Here's how the part is built. I have some questions about the finished solid (model axes, mm). A direction names the side the tool comes from. Round coordinates to 2 decimals unless told otherwise and drop trailing zeros. Write each loop counter-clockwise with the first axis right and the second up, starting at its lowest first coordinate (ties: lowest second). Pieces come first, ordered by that corner, then holes. Notation, with made-up numbers: (-0.75, 77) - (33.25, 77) arc R14 cw to (33.25, 88) - close; hole circle Ø9 at (-9, 76.5). An arc over 180 degrees is marked (long way). One line per item, written item: value. Start each with the question number.
Item 1: If I drill on line 1 (Z direction, x = -3.25, y = 0.75); line 2 (Z direction, x = -3.75, y = 4.25); line 3 (Y direction, x = 0, z = -14.5), over which ranges is the centre line in solid material (lowest first)?
Item 2: For P1, Ø6, axis at x = -4, z = -11.5, coming from the +Y side; P2, Ø1.2, axis at y = -2, z = 17, coming from the +X side; P3, Ø1, axis at x = -0.5, z = 2, coming from the +Y side, each with a flat end and sliding along its axis, tell me the tip position at first contact or that it passes through.
Item 3: Thinking about a two-plate mould opening in X: for faces 1 (the face through (-2.539, -1.947, 9.806)), 2 (the face through (-3, -3, 13.75)), 3 (the face through (-0.75, 0, 17)), 4 (the face through (0, 0, 16.65)), which applies, released by +X, released by -X, zero draft, split by the parting line, or undercut?
Item 4: For faces 5 (the face through (5.96, 1.88, 4.96)), 6 (the face through (3, 0, 18.15)), 7 (the face through (0.75, 0, 17)), 8 (the face through (-2.87, 2.64, -6.6)), 9 (the face through (3, -3, 5.75)), which set-ups out of +Z, -Z, +X, -X, +Y, -Y let a thin tool reach every point of the face, with its end or its side?
Item 5: Imagine slicing it at B-B, the plane x = 0. Please give me the cut outline in (y, z).
Item 6: Imagine slicing it at C-C, the plane y = 0. Please give me the cut outline in (x, z).
Item 7: Imagine slicing it at D-D, the plane z = 10. Please give me the cut outline in (x, y), then the cut area to 3 significant figures.
Item 8: Imagine slicing it at A-A, the plane y = 5. Please give me the cut outline in (x, z).
```python
from build123d import *

# Parameters (mm, degrees)
F2_W     = 1.5
F2_H     = 13
F3_DEPTH = 1.5


with BuildPart() as f1:
    # F0 (on Front) → F1 (revolve)
    with BuildSketch(Plane.XZ):
        Polygon((0, 18.15), (0, -18.15), (3.4, -18.15), (3.9, -17.65), (3.9, 4.15), (6.25, 4.15), (6.25, 5.75), (3.2, 5.75), (3.2, 13.75), (6.25, 13.75), (6.25, 18.15), align=None)
    revolve(axis=Axis((0, 0, 0), (0, 0, 1)))

    # F2 (on face) → F3 (cut)
    with BuildSketch(Plane.XY.offset(18.15)):
        Rectangle(F2_W, F2_H)
    extrude(amount=-F3_DEPTH, mode=Mode.SUBTRACT)


solid = f1.part
```
Values follow:
1. line 1: z = -18.15 to 5.75, 13.75 to 18.15
1. line 2: z = 4.15 to 5.75, 13.75 to 18.15
1. line 3: y = -3.9 to 3.9
2. P1: stops at y = 3.77
2. P2: stops at x = 6.09
2. P3: stops at y = 3.9
3. face 1: split by the parting line
3. face 2: zero draft
3. face 3: undercut
3. face 4: undercut
4. face 5: +Z, -Z
4. face 6: +Z, +X, -X, +Y, -Y
4. face 7: +Z, +Y, -Y
4. face 8: -Z
4. face 9: none
5. outline: (-6.25, 4.15) - (-3.9, 4.15) - (-3.9, -17.65) - (-3.4, -18.15) - (3.4, -18.15) - (3.9, -17.65) - (3.9, 4.15) - (6.25, 4.15) - (6.25, 5.75) - (3.2, 5.75) - (3.2, 13.75) - (6.25, 13.75) - (6.25, 16.65) - (-6.25, 16.65) - (-6.25, 13.75) - (-3.2, 13.75) - (-3.2, 5.75) - (-6.25, 5.75) - close
6. outline: (-6.25, 4.15) - (-3.9, 4.15) - (-3.9, -17.65) - (-3.4, -18.15) - (3.4, -18.15) - (3.9, -17.65) - (3.9, 4.15) - (6.25, 4.15) - (6.25, 5.75) - (3.2, 5.75) - (3.2, 13.75) - (6.25, 13.75) - (6.25, 18.15) - (0.75, 18.15) - (0.75, 16.65) - (-0.75, 16.65) - (-0.75, 18.15) - (-6.25, 18.15) - (-6.25, 13.75) - (-3.2, 13.75) - (-3.2, 5.75) - (-6.25, 5.75) - close
7. outline: circle Ø6.4 at (0, 0)
7. area: 32.2 mm^2
8. outline: (-3.75, 4.15) - (3.75, 4.15) - (3.75, 5.75) - (-3.75, 5.75) - close; (-3.75, 13.75) - (3.75, 13.75) - (3.75, 18.15) - (0.75, 18.15) - (0.75, 16.65) - (-0.75, 16.65) - (-0.75, 18.15) - (-3.75, 18.15) - close
